Check sheet for the modelled part. Datum: model origin and axes. Units: mm. Coordinates: 2 decimals unless noted, no trailing zeros. Loops run counter-clockwise (first coordinate to the right, second up) from the corner with the lowest first, then second, coordinate; pieces in that order, holes last.
```python
from build123d import *

# Parameters (mm, degrees)
SKETCH1_W           = 60.5
SKETCH1_H           = 105
BOSS_EXTRUDE1_DEPTH = 3
SKETCH2_R           = 0.9
CUT_EXTRUDE1_DEPTH  = 3
SKETCH4_R           = 0.9
CUT_EXTRUDE2_DEPTH  = 3
SKETCH5_W           = 15
SKETCH5_H           = 7
CUT_EXTRUDE3_DEPTH  = 3
CUT_EXTRUDE4_DEPTH  = 3


with BuildPart() as part:
    # Sketch1 → Boss-Extrude1 (new body)
    with BuildSketch(Plane(origin=(0, 0, 0), x_dir=(1, 0, 0), z_dir=(0, 1, 0))):
        Rectangle(SKETCH1_W, SKETCH1_H)
    extrude(amount=BOSS_EXTRUDE1_DEPTH)

    # Sketch2 → Cut-Extrude1 (cut)
    with BuildSketch(Plane(origin=(0, 3, 0), x_dir=(1, 0, 0), z_dir=(0, 1, 0))):
        with Locations((-28.25, 49.5)):
            Circle(SKETCH2_R)
        with Locations((28.25, 49.5)):
            Circle(SKETCH2_R)
    extrude(amount=-CUT_EXTRUDE1_DEPTH, mode=Mode.SUBTRACT)

    # Sketch4 → Cut-Extrude2 (cut)
    with BuildSketch(Plane(origin=(0, 3, 0), x_dir=(1, 0, 0), z_dir=(0, 1, 0))):
        with Locations((-28.25, -49.5)):
            Circle(SKETCH4_R)
        with Locations((28.25, -49.5)):
            Circle(SKETCH4_R)
    extrude(amount=-CUT_EXTRUDE2_DEPTH, mode=Mode.SUBTRACT)

    # Sketch5 → Cut-Extrude3 (cut)
    with BuildSketch(Plane(origin=(0, 3, 0), x_dir=(1, 0, 0), z_dir=(0, 1, 0))):
        with Locations((18.75, -5)):
            Rectangle(SKETCH5_W, SKETCH5_H)
    extrude(amount=-CUT_EXTRUDE3_DEPTH, mode=Mode.SUBTRACT)

    # Sketch6 → Cut-Extrude4 (cut)
    with BuildSketch(Plane(origin=(0, 3, 0), x_dir=(1, 0, 0), z_dir=(0, 1, 0))):
        with BuildLine():
            ThreePointArc((23.75286773, 38.214829885), (-0.024201003, 48.23018139), (-23.465757765, 37.452905298))
            ThreePointArc((-23.465757765, 37.452905298), (-23.337849069, 35.335444704), (-21.220388476, 35.4633534))
            ThreePointArc((-21.220388476, 35.4633534), (0.024201003, 45.230571874), (21.572857921, 36.153869615))
            ThreePointArc((21.572857921, 36.153869615), (23.693342961, 36.094344845), (23.75286773, 38.214829885))
        make_face()
        with BuildLine():
            ThreePointArc((23.75286773, 28.214829885), (-0.024201003, 38.23018139), (-23.465757765, 27.452905298))
            ThreePointArc((-23.465757765, 27.452905298), (-23.337849069, 25.335444704), (-21.220388476, 25.4633534))
            ThreePointArc((-21.220388476, 25.4633534), (0.024201003, 35.230571874), (21.572857921, 26.153869615))
            ThreePointArc((21.572857921, 26.153869615), (23.693342961, 26.094344845), (23.75286773, 28.214829885))
        make_face()
        with BuildLine():
            ThreePointArc((23.75286773, 18.214829885), (-0.024201003, 28.23018139), (-23.465757765, 17.452905298))
            ThreePointArc((-23.465757765, 17.452905298), (-23.337849069, 15.335444704), (-21.220388476, 15.4633534))
            ThreePointArc((-21.220388476, 15.4633534), (0.024201003, 25.230571874), (21.572857921, 16.153869615))
            ThreePointArc((21.572857921, 16.153869615), (23.693342961, 16.094344845), (23.75286773, 18.214829885))
        make_face()
        with BuildLine():
            ThreePointArc((23.75286773, 8.214829885), (-0.024201003, 18.23018139), (-23.465757765, 7.452905298))
            ThreePointArc((-23.465757765, 7.452905298), (-23.337849069, 5.335444704), (-21.220388476, 5.4633534))
            ThreePointArc((-21.220388476, 5.4633534), (0.024201003, 15.230571874), (21.572857921, 6.153869615))
            ThreePointArc((21.572857921, 6.153869615), (23.693342961, 6.094344845), (23.75286773, 8.214829885))
        make_face()
        with BuildLine():
            ThreePointArc((23.75286773, -1.785170115), (-0.024201003, 8.23018139), (-23.465757765, -2.547094702))
            ThreePointArc((-23.465757765, -2.547094702), (-23.337849069, -4.664555296), (-21.220388476, -4.5366466))
            ThreePointArc((-21.220388476, -4.5366466), (0.024201003, 5.230571874), (21.572857921, -3.846130385))
            ThreePointArc((21.572857921, -3.846130385), (23.693342961, -3.905655155), (23.75286773, -1.785170115))
        make_face()
        with BuildLine():
            ThreePointArc((23.75286773, -11.785170115), (-0.024201003, -1.76981861), (-23.465757765, -12.547094702))
            ThreePointArc((-23.465757765, -12.547094702), (-23.337849069, -14.664555296), (-21.220388476, -14.5366466))
            ThreePointArc((-21.220388476, -14.5366466), (0.024201003, -4.769428126), (21.572857921, -13.846130385))
            ThreePointArc((21.572857921, -13.846130385), (23.693342961, -13.905655155), (23.75286773, -11.785170115))
        make_face()
        with BuildLine():
            ThreePointArc((23.75286773, -21.785170115), (-0.024201003, -11.76981861), (-23.465757765, -22.547094702))
            ThreePointArc((-23.465757765, -22.547094702), (-23.337849069, -24.664555296), (-21.220388476, -24.5366466))
            ThreePointArc((-21.220388476, -24.5366466), (0.024201003, -14.769428126), (21.572857921, -23.846130385))
            ThreePointArc((21.572857921, -23.846130385), (23.693342961, -23.905655155), (23.75286773, -21.785170115))
        make_face()
        with BuildLine():
            ThreePointArc((23.75286773, -31.785170115), (-0.024201003, -21.76981861), (-23.465757765, -32.547094702))
            ThreePointArc((-23.465757765, -32.547094702), (-23.337849069, -34.664555296), (-21.220388476, -34.5366466))
            ThreePointArc((-21.220388476, -34.5366466), (0.024201003, -24.769428126), (21.572857921, -33.846130385))
            ThreePointArc((21.572857921, -33.846130385), (23.693342961, -33.905655155), (23.75286773, -31.785170115))
        make_face()
        with BuildLine():
            ThreePointArc((23.75286773, -41.785170115), (-0.024201003, -31.76981861), (-23.465757765, -42.547094702))
            ThreePointArc((-23.465757765, -42.547094702), (-23.337849069, -44.664555296), (-21.220388476, -44.5366466))
            ThreePointArc((-21.220388476, -44.5366466), (0.024201003, -34.769428126), (21.572857921, -43.846130385))
            ThreePointArc((21.572857921, -43.846130385), (23.693342961, -43.905655155), (23.75286773, -41.785170115))
        make_face()
    extrude(amount=-CUT_EXTRUDE4_DEPTH, mode=Mode.SUBTRACT)


solid = part.part
```
1) Mould release check, pull along Z, two halves, no side actions. Record for faces 1 (the flat face through (0, 3, -1)), 2 (the cylindrical face through (23.7, 1.5, -26.1)), 3 (the flat face through (0, 1, 52.5)): +Z half, -Z half, draft (parallel to the pull), parting line (faces both ways), or undercut.
Answer sheet:
face 1: draft
face 2: undercut
face 3: +Z half
2) Section check B-B on x = -4.5. Give the number of separate pieces and of enclosed holes in the cut face, plus the area to 3 significant figures.
Answer sheet:
separate pieces: 10
enclosed holes: 0
area: 233 mm2
3) Scan lines: line 1 (X direction, y = 1.8, z = 49.5); line 2 (Z direction, x = 28.25, y = 1.45); line 3 (X direction, y = 1, z = 9). Record each from-to range of solid material in increasing order.
Answer sheet:
line 1: x = -30.25 to -29.15, -27.35 to 27.35, 29.15 to 30.25
line 2: z = -52.5 to -50.4, -48.6 to 48.6, 50.4 to 52.5
line 3: x = -30.25 to -19.78, -14.6 to 15.58, 20.76 to 30.25
4) Section check A-A on z = 17. Enter the section's corners in (x, y).
Answer sheet:
outline: (-30.25, 0) - (-17.05, 0) - (-17.05, 3) - (-30.25, 3) - close; (-10.67, 0) - (11.66, 0) - (11.66, 3) - (-10.67, 3) - close; (18.03, 0) - (30.25, 0) - (30.25, 3) - (18.03, 3) - close
